Could you check a few things on this model? Use its own coordinates, in mm. Face numbers are marked on the shaded views. A direction names the side the tool comes from. Round coordinates to 2 decimals unless told otherwise and drop trailing zeros. Loops run counter-clockwise (first coordinate to the right, second up) from the corner with the lowest first, then second, coordinate; pieces in that order, holes last. Notation, with made-up numbers: (-37, 26.5) - (19, 26.5) arc R20 ccw to (19, 30.5) - close; hole circle Ø7 at (55.25, 38.25). An arc over 180 degrees is marked (long way). Use one line per item in the form item = value.
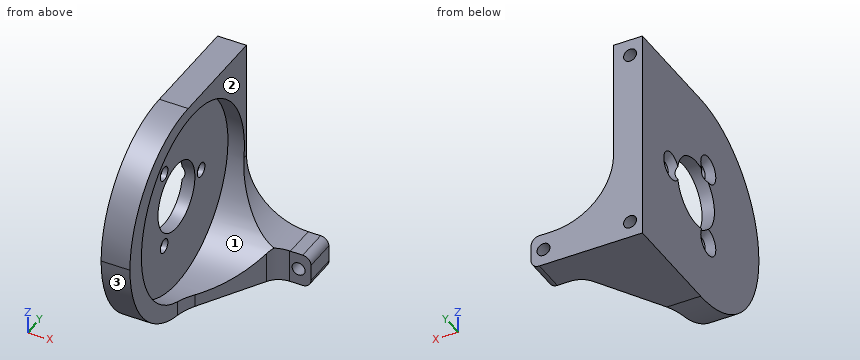
```python
from build123d import *
from OCP.BRepFilletAPI import BRepFilletAPI_MakeChamfer

# Parameters (mm, degrees)
ESBO_O1_W                                      = 52
ESBO_O1_H                                      = 52
RESSALTO_EXTRUS_O1_DEPTH                       = 7
ESBO_O2_R                                      = 8.25
CORTE_EXTRUS_O1_DEPTH                          = 74.87151007
ESCAREADO_PARA_SFHCS_M31_D                     = 3.4
ESCAREADO_PARA_SFHCS_M31_CSINK_D               = 6.72
ESCAREADO_PARA_SFHCS_M31_CSINK_ANGLE           = 90
PADR_OCIRCULAR1_COUNT                          = 3
ESBO_O27_R                                     = 23
CORTE_EXTRUS_O5_DEPTH                          = 4
FILETE1_R                                      = 26
FURO_ROSCADO_PARA_CONDU_TE_DE_M3X0_51_AT_COUNT = 2
FURO_ROSCADO_PARA_CONDU_TE_DE_M3X0_51_AT_PITCH = 44
ESBO_O35_W                                     = 20
ESBO_O35_H                                     = 52
RESSALTO_EXTRUS_O2_DEPTH                       = 8
ESBO_O37_R                                     = 23
CORTE_EXTRUS_O6_DEPTH                          = 77.210235533
CHANFRO1_SIZE                                  = 12
CHANFRO1_SIZE2                                 = 20
FILETE2_R                                      = 10
FILETE3_R                                      = 5
CORTE_EXTRUS_O7_REACH                          = 80.339
ESBO_O39_W                                     = 20
ESBO_O39_H                                     = 36
FILETE5_R                                      = 15
FILETE6_R                                      = 2
CORTE_EXTRUS_O8_REACH                          = 80.339
ESBO_O40_W                                     = 32.243724172
ESBO_O40_H                                     = 53.230333596


with BuildPart() as part:
    # Esboço1 → Ressalto-extrusão1 (new body)
    with BuildSketch(Plane(origin=(0, 0, 0), x_dir=(0, 0, -1), z_dir=(1, 0, 0))):
        with Locations((26, 26)):
            Rectangle(ESBO_O1_W, ESBO_O1_H)
    extrude(amount=RESSALTO_EXTRUS_O1_DEPTH)

    # Esboço2 → Corte-extrusão1 (cut, through all)
    with BuildSketch(Plane.ZY):
        with Locations((-26, 28.1)):
            Circle(ESBO_O2_R)
    extrude(amount=-CORTE_EXTRUS_O1_DEPTH, mode=Mode.SUBTRACT)

    # Escareado para SFHCS M31 (through all)
    with Locations(Plane.ZY):
        with Locations((-26, 39.1)):
            escareado_para_sfhcs_m31 = CounterSinkHole(ESCAREADO_PARA_SFHCS_M31_D / 2, ESCAREADO_PARA_SFHCS_M31_CSINK_D / 2, counter_sink_angle=ESCAREADO_PARA_SFHCS_M31_CSINK_ANGLE)

    # PadrãoCircular1: Escareado para SFHCS M31 ×3 about axis
    padr_ocircular1_axis = Axis((0, 28.1, -26), (1, 0, 0))
    for i in range(1, PADR_OCIRCULAR1_COUNT):
        add(escareado_para_sfhcs_m31.rotate(padr_ocircular1_axis, i * 360 / PADR_OCIRCULAR1_COUNT), mode=Mode.SUBTRACT)

    # Esboço27 → Corte-extrusão5 (cut)
    with BuildSketch(Plane(origin=(7, 0, 0), x_dir=(0, 0, -1), z_dir=(1, 0, 0))):
        with Locations((26, 28.1)):
            Circle(ESBO_O27_R)
    extrude(amount=-CORTE_EXTRUS_O5_DEPTH, mode=Mode.SUBTRACT)

    # Filete1
    filete1_edges = [part.edges().sort_by_distance(p)[0] for p in [
        (3.5, 0, -52),
        (3.5, 0, 0),
    ]]
    fillet(filete1_edges, radius=FILETE1_R - 0.0001)  # a hair under: the kernel refuses the full size

    # Esboço34 → Furo roscado para conduíte de M3x0.51 (revolve, cut)
    with BuildSketch(Plane(origin=(3, 52, -48), x_dir=(0, 0, 1), z_dir=(1, 0, 0))):
        Polygon((0, 0), (0, 10.946355475), (1.575, 10), (1.575, 0), align=None)
    furo_roscado_para_condu_te_de_m3x0_51 = revolve(axis=Axis((3, 58.35, -48), (0, -1, 0)), mode=Mode.SUBTRACT)

    # Furo roscado para conduíte de M3x0.51 at: Furo roscado para conduíte de M3x0.51 ×2
    with Locations(*[(0, 0, i * FURO_ROSCADO_PARA_CONDU_TE_DE_M3X0_51_AT_PITCH) for i in range(1, FURO_ROSCADO_PARA_CONDU_TE_DE_M3X0_51_AT_COUNT)]):
        add(furo_roscado_para_condu_te_de_m3x0_51, mode=Mode.SUBTRACT)

    # Esboço35 → Ressalto-extrusão2 (add)
    with BuildSketch(Plane(origin=(0, 52, 0), x_dir=(1, 0, 0), z_dir=(0, 1, 0))):
        with Locations((17, 26)):
            Rectangle(ESBO_O35_W, ESBO_O35_H)
    extrude(amount=-RESSALTO_EXTRUS_O2_DEPTH)

    # Esboço37 → Corte-extrusão6 (cut, through all)
    with BuildSketch(Plane(origin=(7, 0, 0), x_dir=(0, 0, -1), z_dir=(1, 0, 0))):
        with Locations((26, 28.1)):
            Circle(ESBO_O37_R)
    extrude(amount=CORTE_EXTRUS_O6_DEPTH, mode=Mode.SUBTRACT)

    # Chanfro1: one chamfer whose edges measure the first distance from different faces: ONE call of the kernel's chamfer builder (chamfer() names one face for all edges)
    chanfro1_edges_1 = [part.edges().sort_by_distance(p)[0] for p in [
        (7, 44, -47.309482535),
    ]]
    chanfro1_side_1 = [part.faces().sort_by_distance(p)[0] for p in [
        (17, 44, -47.309482535),
    ]]
    chanfro1_edges_2 = [part.edges().sort_by_distance(p)[0] for p in [
        (7, 44, -4.690517465),
    ]]
    chanfro1_side_2 = [part.faces().sort_by_distance(p)[0] for p in [
        (17, 44, -4.690517465),
    ]]
    chanfro1 = BRepFilletAPI_MakeChamfer(part.part.solid().wrapped)
    for e in chanfro1_edges_1:
        chanfro1.Add(CHANFRO1_SIZE, CHANFRO1_SIZE2, e.wrapped, chanfro1_side_1[0].wrapped)  # the first distance lies on this face
    for e in chanfro1_edges_2:
        chanfro1.Add(CHANFRO1_SIZE, CHANFRO1_SIZE2, e.wrapped, chanfro1_side_2[0].wrapped)  # the first distance lies on this face
    add(Compound.cast(chanfro1.Shape()), mode=Mode.REPLACE)

    # Filete2
    filete2_edges = [part.edges().sort_by_distance(p)[0] for p in [
        (7, 24, -1.722707367),
        (7, 24, -50.277292633),
    ]]
    fillet(filete2_edges, radius=FILETE2_R)

    # Filete3
    filete3_edges = [part.edges().sort_by_distance(p)[0] for p in [
        (19, 44, -4.690517465),
        (19, 44, -47.309482535),
    ]]
    fillet(filete3_edges, radius=FILETE3_R)

    # Espelhar1: Furo roscado para conduíte de M3x0.51 across plane
    add(furo_roscado_para_condu_te_de_m3x0_51.mirror(Plane.ZY.offset(-13.5)), mode=Mode.SUBTRACT)

    # Espelhar1 copy 1 sketch → Espelhar1 copy 1 (revolve, cut)
    with BuildSketch(Plane(origin=(24, 52, -4), x_dir=(0, 0, 1), z_dir=(-1, 0, 0))):
        Polygon((0, 0), (0, -10.946355475), (1.575, -10), (1.575, 0), align=None)
    revolve(axis=Axis((24, 58.35, -4), (0, 1, 0)), mode=Mode.SUBTRACT)

    # Esboço39 → Corte-extrusão7 (cut, up to next)
    with BuildSketch(Plane(origin=(0, 52, 0), x_dir=(1, 0, 0), z_dir=(0, 1, 0)), mode=Mode.PRIVATE) as corte_extrus_o7_sk1:
        with Locations((17, 26)):
            Rectangle(ESBO_O39_W, ESBO_O39_H)
    corte_extrus_o7_tool1 = extrude(corte_extrus_o7_sk1.sketch, amount=-CORTE_EXTRUS_O7_REACH, mode=Mode.PRIVATE) & part.part
    add(corte_extrus_o7_tool1.solids().sort_by_distance((17, 52, -26))[0], mode=Mode.SUBTRACT)

    # Filete5
    filete5_edges = [part.edges().sort_by_distance(p)[0] for p in [
        (7, 47.208910532, -44),
        (7, 47.208910532, -8),
    ]]
    fillet(filete5_edges, radius=FILETE5_R)

    # Filete6
    filete6_edges = [part.edges().sort_by_distance(p)[0] for p in [
        (27, 48, -44),
        (27, 48, -8),
        (27, 48, -52),
        (27, 48, 0),
    ]]
    fillet(filete6_edges, radius=FILETE6_R)

    # Esboço40 → Corte-extrusão8 (cut, up to next)
    with BuildSketch(Plane.XY, mode=Mode.PRIVATE) as corte_extrus_o8_sk1:
        with Locations((23.121862086, 26.615166798)):
            Rectangle(ESBO_O40_W, ESBO_O40_H)
    corte_extrus_o8_tool1 = extrude(corte_extrus_o8_sk1.sketch, amount=-CORTE_EXTRUS_O8_REACH, mode=Mode.PRIVATE) & part.part
    add(corte_extrus_o8_tool1.solids().sort_by_distance((23.121862, 26.615167, 0))[0], mode=Mode.SUBTRACT)


solid = part.part
```
1. If we section it at D-D, the plane y = 17: Write out the boundary of the cut face in (x, z).
Solution:
outline = (0, -50.39) - (7, -50.39) - (7, -46.14) - (3, -46.14) - (3, -5.86) - (7, -5.86) - (7, -1.61) - (0, -1.61) - close
2. On a 3-axis mill with a long thin cutter (end or side, diameter ignored), from which of +Z, -Z, +X, -X, +Y, -Y can I reach the whole of each face in a straight line? I mean the marked faces 1, 2 and 3. Say none if no direction works.
Solution:
face_1 = +X
face_2 = +Z, +X, -Y
face_3 = -Z, +X, -X, -Y
3. For P1, Ø1.9, axis at x = 24, z = -48, coming from the -Y side; P2, Ø4.5, axis at y = 22.6, z = -35.53, coming from the -X side; P3, Ø2, axis at x = 10, z = -42, coming from the -Y side; P4, Ø4, axis at x = 25, z = -47.5, coming from the -Y side, each with a flat end and sliding along its axis, tell me the tip position at first contact or that it passes through.
Solution:
P1 = through
P2 = 1.11
P3 = 43.59
P4 = 44
4. If we section it at C-C, the plane y = 33.5: Write out the boundary of the cut face in (x, z).
Solution:
outline = (0, -52) - (12.7, -52) - (12.7, -48.36) - (3, -48.36) - (3, -32.24) - (0, -32.24) - close; (0, -19.76) - (3, -19.76) - (3, -3.64) - (7, -3.64) - (7, 0) - (0, 0) - close
5. If we section it at A-A, the plane x = 24: Write out the boundary of the cut face in (y, z) (3 decimals).
Solution:
outline = (44, -52) - (52, -52) - (52, -49.575) - (44, -49.575) - close; (44, -46.425) - (52, -46.425) - (52, -44) - (44, -44) - close
6. Please list where these lines run through material, in increasing order: line 1 along Y through (x, z) = (2, -26); line 2 along X through (y, z) = (47.25, -48) (3 decimals); line 3 along X through (y, z) = (10.5, -8.5).
Solution:
line_1 = 0 to 19.85, 36.35 to 37.4, 40.8 to 52
line_2 = 0 to 1.425, 4.575 to 22.425, 25.575 to 27
line_3 = 0 to 7
7. If we section it at B-B, the plane y = 28.1: Write out the boundary of the cut face in (x, z).
Solution:
outline = (0, -52) - (9.46, -52) - (9.46, -49) - (3, -49) - (3, -34.25) - (0, -34.25) - close; (0, -17.75) - (3, -17.75) - (3, -3) - (7, -3) - (7, 0) - (0, 0) - close
